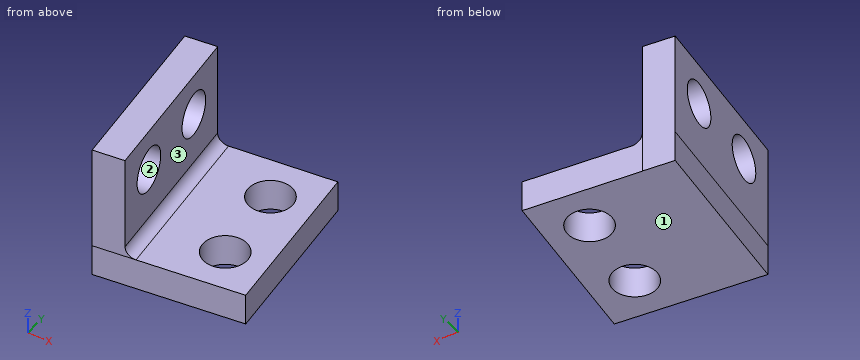
from build123d import *

# Parameters (mm, degrees)
SKETCH1_R           = 2.1
BOSS_EXTRUDE1_DEPTH = 3
SKETCH3_W           = 13
SKETCH3_H           = 16.5
SKETCH3_R           = 2.1
BOSS_EXTRUDE2_DEPTH = 3
FILLET1_R           = 1


with BuildPart() as part:
    # Sketch1 → Boss-Extrude1 (new body)
    with BuildSketch(Plane.XY):
        Polygon((-105, 44.736808962), (-103.35, 28.31951625), (-89.420175881, 29.71951625), (-91.061152102, 46.043912356), align=None)
        with Locations((-94.622025059, 41.474945451)):
            Circle(SKETCH1_R, mode=Mode.SUBTRACT)
        with Locations((-93.848562649, 33.512423495)):
            Circle(SKETCH1_R, mode=Mode.SUBTRACT)
    extrude(amount=BOSS_EXTRUDE1_DEPTH)

    # Sketch3 → Boss-Extrude2 (add)
    with BuildSketch(Plane(origin=(-99.498743711, -10, 0), x_dir=(0, 0, 1), z_dir=(-0.9949874371066202, -0.09999999999999917, 0))):
        with Locations((6.5, 46.762562893)):
            Rectangle(SKETCH3_W, SKETCH3_H)
        with Locations(Location((9, 42.762562893, 0), (0, 0, 270))):
            Circle(SKETCH3_R, mode=Mode.SUBTRACT)
        with Locations(Location((9, 50.762562893, 0), (0, 0, 270))):
            Circle(SKETCH3_R, mode=Mode.SUBTRACT)
    extrude(amount=-BOSS_EXTRUDE2_DEPTH)

    # Fillet1
    fillet1_edges = [part.edges().sort_by_distance(p)[0] for p in [
        (-101.189037666, 36.81821251, 3),
    ]]
    fillet(fillet1_edges, radius=FILLET1_R)


solid = part.part
CAD build for the part. Positions are in the model's coordinates, mm. Face numbers are marked on the shaded views. Round coordinates to 2 decimals unless told otherwise and drop trailing zeros. Write each loop counter-clockwise with the first axis right and the second up, starting at its lowest first coordinate (ties: lowest second). Pieces come first, ordered by that corner, then holes.
(1) Slice it at C-C, the plane z = 5.5. Write the cut outline in (x, y).
(2) Mould opens along Z. For the marked faces 1, 2 and 3 say: pulls with the +Z half, pulls with the -Z half, needs draft (parallel to the pull), parting line crosses it, or undercut.
(3) Slice it at D-D, the plane y = 33.75. Count the separate pieces of the cut face and the enclosed holes in it, and give its area (3 significant figures).
(4) Drop flat-ended pins along their axis: P1, Ø6, axis at x = -97.5, z = 7, coming from the -Y side; P2, Ø5, axis at y = 41.5, z = 5, coming from the -X side; P3, Ø1.5, axis at y = 38, z = 6.5, coming from the -X side; P4, Ø3, axis at x = -93.5, y = 33.5, coming from the +Z side. Give the stop position or say it passes through.
(5) Slice it at A-A, the plane x = -92.25. Write the cut outline in (y, z), and give its area (3 significant figures).
(6) Slice it at B-B, the plane z = 9.25. Write the cut outline in (x, y).
(7) Probe line 1 along Z through (x, y) = (-98.25, 33); line 2 along X through (y, z) = (40.25, 2.75); line 3 along X through (y, z) = (43.5, 6.5). List the from-to ranges inside material, lowest first.
From the geometry:
1. outline: (-105, 44.74) - (-103.35, 28.32) - (-100.37, 28.62) - (-102.02, 45.04) - close
2. face 1: pulls with the -Z half
2. face 2: undercut
2. face 3: needs draft
3. separate pieces: 3
3. enclosed holes: 0
3. area: 49.1 mm2
4. P1: stops at y = 28.61
4. P2: stops at x = -104.93
4. P3: stops at x = -104.4
4. P4: passes through
5. outline: (29.44, 0) - (32.15, 0) - (32.15, 3) - (29.44, 3) - close; (34.87, 0) - (45.93, 0) - (45.93, 3) - (34.87, 3) - close
5. area: 41.3 mm2
6. outline: (-105, 44.74) - (-104.78, 42.58) - (-101.8, 42.88) - (-102.02, 45.04) - close; (-104.37, 38.43) - (-103.98, 34.62) - (-101, 34.92) - (-101.38, 38.73) - close; (-103.57, 30.47) - (-103.35, 28.32) - (-100.37, 28.62) - (-100.58, 30.77) - close
7. line 1: z = 0 to 3
7. line 2: x = -104.55 to -96.33, -92.92 to -90.48
7. line 3: x = -104.88 to -101.86
